from build123d import *

# Parameters (mm, degrees)
EXTRUDE_1_DEPTH = 15.5
SHELL_1_T       = -2


with BuildPart() as part:
    # Эскиз2 → Бобышка-Вытянуть1 (new body)
    with BuildSketch(Plane(origin=(0, 0, 0), x_dir=(1, 0, 0), z_dir=(0, 1, 0))):
        with BuildLine():
            Line((-7, 0), (-76, 0))
            ThreePointArc((-76, 0), (-80.949747468, 2.050252532), (-83, 7))
            Line((-83, 7), (-83, 175))
            ThreePointArc((-83, 175), (-80.949747468, 179.949747468), (-76, 182))
            Line((-76, 182), (-7, 182))
            ThreePointArc((-7, 182), (-2.050252532, 179.949747468), (0, 175))
            Line((0, 175), (0, 7))
            ThreePointArc((0, 7), (-2.050252532, 2.050252532), (-7, 0))
        make_face()
    extrude(amount=EXTRUDE_1_DEPTH)

    # Оболочка1
    shell_1_openings = [part.faces().sort_by_distance(p)[0] for p in [
        (-41.5, 0, -91),
    ]]
    offset(amount=SHELL_1_T, openings=shell_1_openings, kind=Kind.INTERSECTION)


solid = part.part
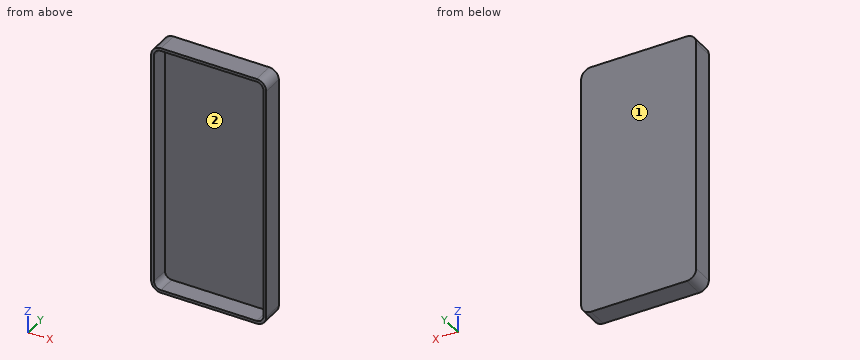
Read the model definition and answer for the solid it produces. Units are mm, in the model's axes. Face numbers are marked on the shaded views. Round coordinates to 2 decimals unless told otherwise and drop trailing zeros. Write each loop counter-clockwise with the first axis right and the second up, starting at its lowest first coordinate (ties: lowest second). Pieces come first, ordered by that corner, then holes. Notation, with made-up numbers: (48.5, -21.5) - (69.5, -21.5) arc R27 ccw to (69.5, 7.5) - close; hole circle Ø5 at (47, 3.25). An arc over 180 degrees is marked (long way). One line per question, with ' | ' between items. Start each with the question number.
1. Section A-A (y = 7.75) is taken. Determine the outline of the cut face in (x, z), and give its area (3 significant figures).
2. Section C-C (x = -24.5) is taken. Determine the outline of the cut face in (y, z), and give its area (3 significant figures).
3. For a pull along X with two mould halves and no side action, classify the marked faces 1 and 2 as +X half, -X half, draft (parallel to the pull), parting line (faces both ways), or undercut.
4. Section B-B (z = -99.5) is taken. Determine the outline of the cut face in (x, y).
5. This flat-tipped pin is pushed along its axis until it touches: pin 1 (1.5 mm diameter, centred on x = -35.5, z = -26.5, fed in from -Y). Where does it stop, or does it pass through?
6. Find the intervals of material crossed by probe 1 along Z at (x, y) = (-64.5, 13); probe 2 along X at (y, z) = (8.75, -151); probe 3 along Y at (x, z) = (-27.5, -32), in increasing order. Write a range as [from, to].
Filled in:
1) outline: (-83, -175) arc R7 ccw to (-76, -182) - (-7, -182) arc R7 ccw to (0, -175) - (0, -7) arc R7 ccw to (-7, 0) - (-76, 0) arc R7 ccw to (-83, -7) - close; hole (-81, -175) arc R5 ccw to (-76, -180) - (-7, -180) arc R5 ccw to (-2, -175) - (-2, -7) arc R5 ccw to (-7, -2) - (-76, -2) arc R5 ccw to (-81, -7) - close | area: 1,020 mm²
2) outline: (0, -182) - (15.5, -182) - (15.5, 0) - (0, 0) - (0, -2) - (13.5, -2) - (13.5, -180) - (0, -180) - close | area: 418 mm²
3) face 1: draft | face 2: undercut
4) outline: (-83, 0) - (-81, 0) - (-81, 13.5) - (-2, 13.5) - (-2, 0) - (0, 0) - (0, 15.5) - (-83, 15.5) - close
5) pin 1: y = 13.5
6) probe 1: [-182, -180], [-2, 0] | probe 2: [-83, -81], [-2, 0] | probe 3: [13.5, 15.5]
